from build123d import *

# Parameters (mm, degrees)
SKETCH_R           = 0.65
PAD_DEPTH          = 5
SKETCH001_W        = 19.2
SKETCH001_H        = 6.7
SKETCH001_W_2      = 15.2
SKETCH001_H_2      = 2.7
SKETCH001_W_3      = 6.7
SKETCH001_H_3      = 19.2
SKETCH001_W_4      = 2.7
SKETCH001_H_4      = 15.2
PAD001_DEPTH       = 5
POLARPATTERN_COUNT = 4
SKETCH002_W        = 87.84
SKETCH002_H        = 87.84
POCKET_DEPTH       = 5
SKETCH003_W        = 186.050454
SKETCH003_H        = 194.116951
SKETCH003_W_2      = 101.24
SKETCH003_H_2      = 101.24
POCKET001_DEPTH    = 5
CHAMFER_SIZE       = 5
CHAMFER001_SIZE    = 2


with BuildPart() as part:
    # Sketch → Pad (new body)
    with BuildSketch(Plane.XY):
        Polygon((-52.00016, -52.00016), (0, -52.00016), (0, -42.00016), (-34.929092, -42.00016), (0, -7.071068), (0, 0), (-7.071068, 0), (-42.00016, -34.929092), (-42.00016, 0), (-52.00016, 0), align=None)
        with Locations((-47.00016, -47.00016)):
            Circle(SKETCH_R, mode=Mode.SUBTRACT)
        with Locations((-26.67, -26.67)):
            Circle(SKETCH_R, mode=Mode.SUBTRACT)
    pad = extrude(amount=PAD_DEPTH)

    # Sketch001 (on Face14 of Pad) → Pad001 (join)
    with BuildSketch(Plane.XY.offset(5)):
        with Locations((-26.67, -47.27)):
            Rectangle(SKETCH001_W, SKETCH001_H)
        with Locations((-26.67, -47.27)):
            Rectangle(SKETCH001_W_2, SKETCH001_H_2, mode=Mode.SUBTRACT)
        with Locations((-47.27, -26.67)):
            Rectangle(SKETCH001_W_3, SKETCH001_H_3)
        with Locations((-47.27, -26.67)):
            Rectangle(SKETCH001_W_4, SKETCH001_H_4, mode=Mode.SUBTRACT)
    pad001 = extrude(amount=PAD001_DEPTH)

    # PolarPattern: Pad, Pad001 ×4 about axis
    polarpattern_axis = Axis((0, 0, 0), (0, 0, 1))
    for i in range(1, POLARPATTERN_COUNT):
        add(pad.rotate(polarpattern_axis, i * 360 / POLARPATTERN_COUNT))
        add(pad001.rotate(polarpattern_axis, i * 360 / POLARPATTERN_COUNT))

    # Sketch002 (on Face20 of PolarPattern) → Pocket (cut)
    with BuildSketch(Plane.XY.offset(5)):
        Rectangle(SKETCH002_W, SKETCH002_H)
    extrude(amount=-POCKET_DEPTH, mode=Mode.SUBTRACT)

    # Sketch003 (on Face5 of Pocket) → Pocket001 (cut)
    with BuildSketch(Plane.XY.offset(5)):
        with Locations((-8.059452, 19.223796)):
            Rectangle(SKETCH003_W, SKETCH003_H)
        Rectangle(SKETCH003_W_2, SKETCH003_H_2, mode=Mode.SUBTRACT)
    extrude(amount=-POCKET001_DEPTH, mode=Mode.SUBTRACT)

    # Chamfer
    chamfer_edges = [part.edges().sort_by_distance(p)[0] for p in [
        (43.92, 43.92, 2.5),
        (43.92, -43.92, 2.5),
        (-43.92, -43.92, 2.5),
        (-43.92, 43.92, 2.5),
    ]]
    chamfer(chamfer_edges, length=CHAMFER_SIZE)

    # Chamfer001
    chamfer001_edges = [part.edges().sort_by_distance(p)[0] for p in [
        (17.07, 47.27, 5),
        (-36.27, 47.27, 5),
        (-47.27, 17.07, 5),
        (-47.27, -36.27, 5),
        (-36.27, -47.27, 5),
        (17.07, -47.27, 5),
        (47.27, -36.27, 5),
        (47.27, 17.07, 5),
        (36.27, 47.27, 5),
        (-17.07, 47.27, 5),
        (-47.27, 36.27, 5),
        (-47.27, -17.07, 5),
        (-17.07, -47.27, 5),
        (36.27, -47.27, 5),
        (47.27, -17.07, 5),
        (47.27, 36.27, 5),
    ]]
    chamfer(chamfer001_edges, length=CHAMFER001_SIZE)


solid = part.part
Work out the finished part from the listing and answer in its coordinate system (mm). A direction names the side the tool comes from. Give positions to 0.01 mm unless a question says otherwise; leave off trailing zeros. Loops run counter-clockwise (first coordinate to the right, second up) from the corner with the lowest first, then second, coordinate; pieces in that order, holes last. Notation, with made-up numbers: (47.5, 1) -> (97.5, 1) arc R20 cw to (97.5, 13) -> close; hole circle Ø3 at (44.5, -24). An arc over 180 degrees is marked (long way). Use a Markdown table: item, result. Add a question column.
1. Section A-A on y = 20.5 is taken. Determine the outline of the cut face in (x, z).
2. For faces 4 (the flat face through (47, -19.07, 7)), 5 (the flat face through (49, 27, 10)), determine the directions among +Z, -Z, +X, -X, +Y, -Y from which every point of the face is accessible in a straight line to the end or side of a thin tool.
3. Find the intervals of material crossed by probe 1 along X at (y, z) = (-32, 5.5); probe 2 along X at (y, z) = (14.5, 1.25), in increasing order.
4. Determine the mould class of faces 1 (the flat face through (-44, 45, 5)), 2 (the flat face through (36.27, -47, 8)), 3 (the flat face through (-47, 19.07, 7)) for opening direction X: released by +X, released by -X, zero draft, split by the parting line, or undercut.
5. Section C-C on z = 2 is taken. Determine the outline of the cut face in (x, y).
6. Flat-ended cylindrical pins translate along their axes: pin 1 Ø0.8 at (x, y) = (-47, 24) entering from +Z; pin 2 Ø3.5 at (x, z) = (-48, 8) entering from +Y; pin 3 Ø1.4 at (x, z) = (47, 8.5) entering from +Y. Find the tip coordinate at first contact, or state that the pin passes through.
7. Section B-B on x = 1 is taken. Determine the outline of the cut face in (y, z).
Results below:
| question | item | result |
|---|---|---|
| 1 | outline | (-50.62, 0) -> (-43.92, 0) -> (-43.92, 10) -> (-45.92, 10) -> (-45.92, 5) -> (-48.62, 5) -> (-48.62, 10) -> (-50.62, 10) -> close; (43.92, 0) -> (50.62, 0) -> (50.62, 10) -> (48.62, 10) -> (48.62, 5) -> (45.92, 5) -> (45.92, 10) -> (43.92, 10) -> close |
| 2 | face 4 | +Z |
| 2 | face 5 | +Z, +X, -X, +Y, -Y |
| 3 | probe 1 | x = -50.62 to -48.62, -45.92 to -43.92, 43.92 to 45.92, 48.62 to 50.62 |
| 3 | probe 2 | x = -50.62 to -43.92, 43.92 to 50.62 |
| 4 | face 1 | zero draft |
| 4 | face 2 | released by +X |
| 4 | face 3 | undercut |
| 5 | outline | (-50.62, -50.62) -> (50.62, -50.62) -> (50.62, 50.62) -> (-50.62, 50.62) -> close; hole circle Ø1.3 at (-47, -47); hole circle Ø1.3 at (-47, 47); hole (-43.92, -38.92) -> (-38.92, -43.92) -> (38.92, -43.92) -> (43.92, -38.92) -> (43.92, 38.92) -> (38.92, 43.92) -> (-38.92, 43.92) -> (-43.92, 38.92) -> close; hole circle Ø1.3 at (47, -47); hole circle Ø1.3 at (47, 47) |
| 6 | pin 1 | stops at z = 5 |
| 6 | pin 2 | stops at y = 37.02 |
| 6 | pin 3 | stops at y = 36.27 |
| 7 | outline | (-50.62, 0) -> (-43.92, 0) -> (-43.92, 5) -> (-50.62, 5) -> close; (43.92, 0) -> (50.62, 0) -> (50.62, 5) -> (43.92, 5) -> close |
